The listing builds one solid part. Answer for the finished solid, in the listing's coordinates (mm). Face numbers are marked on the shaded views. A direction names the side the tool comes from. Coordinates: 2 decimals unless noted, no trailing zeros. Write each loop counter-clockwise with the first axis right and the second up, starting at its lowest first coordinate (ties: lowest second). Pieces come first, ordered by that corner, then holes.
(1) The part is cut by section C-C on y = 1.5. Determine the outline of the cut face in (x, z).
(2) The part is cut by section B-B on x = 0. Determine the outline of the cut face in (y, z), plus the area to 3 significant figures.
(3) The part is cut by section A-A on z = 0. Determine the outline of the cut face in (x, y), plus the area to 3 significant figures.
(4) Straight lines are drawn through the part: line 1 (Z direction, x = 28, y = -2.25); line 2 (Z direction, x = -23, y = 1.45); line 3 (Y direction, x = 26.5, z = 0.5). For each, find the intervals that lie inside material, in ascending order.
(5) The part is cut by section D-D on x = 24. Determine the outline of the cut face in (y, z) (3 decimals).
(6) Which of the six approach directions +Z, -Z, +X, -X, +Y, -Y give full straight-line access (tool end or side, diameter ignored) to the marked faces 1 and 2?
(7) Given P1, Ø1, axis at x = -18, z = 14, coming from the -Y side, flat-ended and moving along its own axis, determine where the tip first touches the part or whether it passes through.
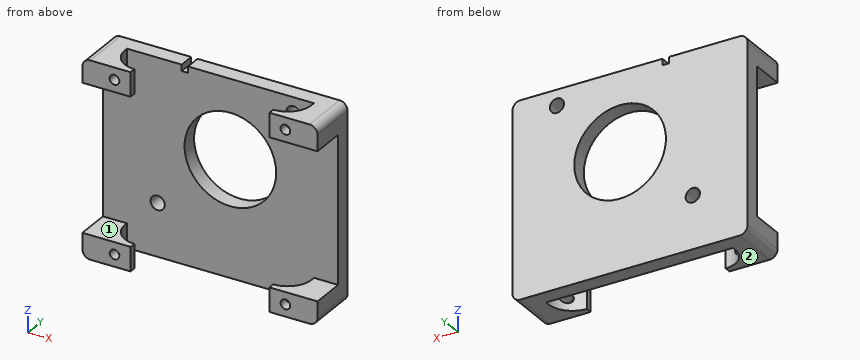
from build123d import *

# Parameters (mm, degrees)
SKETCH1_R           = 14.5
SKETCH1_R_2         = 2.25
BOSS_EXTRUDE1_DEPTH = 5
SKETCH2_W           = 7.62
SKETCH2_H           = 7.62
BOSS_EXTRUDE2_DEPTH = 10.795
SKETCH4_W           = 7.62
SKETCH4_H           = 7.62
SKETCH4_R           = 1.524
BOSS_EXTRUDE3_DEPTH = 2
BOSS_EXTRUDE4_START = -7.62
BOSS_EXTRUDE4_DEPTH = 7.62
BOSS_EXTRUDE5_START = -7.62
BOSS_EXTRUDE5_DEPTH = 7.62
SKETCH4_2_R         = 1.524
CUT_EXTRUDE1_DEPTH  = 10.795
FILLET1_R           = 2.54


with BuildPart() as part:
    # Sketch1 → Boss-Extrude1 (new body)
    with BuildSketch(Plane(origin=(0, 0, 0), x_dir=(1, 0, 0), z_dir=(0, 1, 0))):
        Polygon((-40.324, -25), (-15.4, -25), (-15.4, -23), (-13.4, -23), (-13.4, -25), (34.098, -25), (34.098, 36.722), (-40.324, 36.722), align=None)
        Circle(SKETCH1_R, mode=Mode.SUBTRACT)
        with Locations((-23, 20)):
            Circle(SKETCH1_R_2, mode=Mode.SUBTRACT)
        with Locations((20, -20)):
            Circle(SKETCH1_R_2, mode=Mode.SUBTRACT)
    extrude(amount=BOSS_EXTRUDE1_DEPTH)

    # Sketch2 → Boss-Extrude2 (add)
    with BuildSketch(Plane.XZ):
        with Locations((-36.514, 21.19)):
            Rectangle(SKETCH2_W, SKETCH2_H)
        with Locations((30.288, 21.19)):
            Rectangle(SKETCH2_W, SKETCH2_H)
        with Locations((30.288, -32.912)):
            Rectangle(SKETCH2_W, SKETCH2_H)
        with Locations((-36.514, -32.912)):
            Rectangle(SKETCH2_W, SKETCH2_H)
    extrude(amount=BOSS_EXTRUDE2_DEPTH)

    # Sketch4 → Boss-Extrude3 (add)
    with BuildSketch(Plane.XZ.offset(10.795)):
        with Locations((-28.894, 21.19)):
            Rectangle(SKETCH4_W, SKETCH4_H)
        with Locations((-30.164, 21.19)):
            Circle(SKETCH4_R, mode=Mode.SUBTRACT)
        with Locations((-28.894, -32.912)):
            Rectangle(SKETCH4_W, SKETCH4_H)
        with Locations((-30.164, -32.912)):
            Circle(SKETCH4_R, mode=Mode.SUBTRACT)
        with Locations((22.668, -32.912)):
            Rectangle(SKETCH4_W, SKETCH4_H)
        with Locations((23.938, -32.912)):
            Circle(SKETCH4_R, mode=Mode.SUBTRACT)
        with Locations((22.668, 21.19)):
            Rectangle(SKETCH4_W, SKETCH4_H)
        with Locations((23.938, 21.19)):
            Circle(SKETCH4_R, mode=Mode.SUBTRACT)
    extrude(amount=-BOSS_EXTRUDE3_DEPTH)

    # Sketch5 → Boss-Extrude4 (add)
    with BuildSketch(Plane.XY.offset(25).offset(BOSS_EXTRUDE4_START)):
        with BuildLine():
            Line((-25.084, -8.795), (-32.704, -8.795))
            Line((-32.704, -8.795), (-32.704, -1.175))
            ThreePointArc((-32.704, -1.175), (-30.472153673, -6.563153673), (-25.084, -8.795))
        make_face()
        with BuildLine():
            Line((18.858, -8.795), (26.478, -8.795))
            Line((26.478, -8.795), (26.478, -1.175))
            ThreePointArc((26.478, -1.175), (24.246153673, -6.563153673), (18.858, -8.795))
        make_face()
    extrude(amount=BOSS_EXTRUDE4_DEPTH)

    # Sketch6 → Boss-Extrude5 (add)
    with BuildSketch(Plane(origin=(0, 0, -36.722), x_dir=(-1, 0, 0), z_dir=(0, 0, -1)).offset(BOSS_EXTRUDE5_START)):
        with BuildLine():
            Line((-26.478, -8.795), (-26.478, -1.175))
            ThreePointArc((-26.478, -1.175), (-24.246153673, -6.563153673), (-18.858, -8.795))
            Line((-18.858, -8.795), (-26.478, -8.795))
        make_face()
        with BuildLine():
            Line((32.704, -8.795), (32.704, -1.175))
            ThreePointArc((32.704, -1.175), (30.472153673, -6.563153673), (25.084, -8.795))
            Line((25.084, -8.795), (32.704, -8.795))
        make_face()
    extrude(amount=BOSS_EXTRUDE5_DEPTH)

    # Sketch4<2> → Cut-Extrude1 (cut)
    with BuildSketch(Plane.XZ.offset(10.795)):
        with Locations((23.938, 21.19)):
            Circle(SKETCH4_2_R)
        with Locations((-30.164, -32.912)):
            Circle(SKETCH4_2_R)
        with Locations((-30.164, 21.19)):
            Circle(SKETCH4_2_R)
        with Locations((23.938, -32.912)):
            Circle(SKETCH4_2_R)
    extrude(amount=-CUT_EXTRUDE1_DEPTH, mode=Mode.SUBTRACT)

    # Fillet1
    fillet1_edges = [part.edges().sort_by_distance(p)[0] for p in [
        (-40.324, -2.8975, 25),
        (-40.324, -2.8975, -36.722),
        (34.098, -2.8975, -36.722),
        (34.098, -2.8975, 25),
    ]]
    fillet(fillet1_edges, radius=FILLET1_R)


solid = part.part
Model answer:
1. outline: (-40.32, -34.18) arc R2.54 ccw to (-37.78, -36.72) - (31.56, -36.72) arc R2.54 ccw to (34.1, -34.18) - (34.1, 22.46) arc R2.54 ccw to (31.56, 25) - (-13.4, 25) - (-13.4, 23) - (-15.4, 23) - (-15.4, 25) - (-37.78, 25) arc R2.54 ccw to (-40.32, 22.46) - close; hole circle Ø4.5 at (-23, -20); hole circle Ø29 at (0, 0); hole circle Ø4.5 at (20, 20)
2. outline: (0, -36.72) - (5, -36.72) - (5, -14.5) - (0, -14.5) - close; (0, 14.5) - (5, 14.5) - (5, 25) - (0, 25) - close
2. area: 164 mm2
3. outline: (-40.32, 0) - (-14.5, 0) - (-14.5, 5) - (-40.32, 5) - close; (14.5, 0) - (34.1, 0) - (34.1, 5) - (14.5, 5) - close
3. area: 227 mm2
4. line 1: z = -36.72 to -29.1, 17.38 to 25
4. line 2: z = -36.72 to -22.25, -17.75 to 25
4. line 3: y = 0 to 5
5. outline: (-10.795, -36.722) - (-6.799, -36.722) - (-6.799, -34.435) - (-10.795, -34.435) - close; (-10.795, -31.389) - (-6.799, -31.389) - (-6.799, -29.102) - (-10.795, -29.102) - close; (-10.795, 17.38) - (-6.799, 17.38) - (-6.799, 19.667) - (-10.795, 19.667) - close; (-10.795, 22.713) - (-6.799, 22.713) - (-6.799, 25) - (-10.795, 25) - close; (0, -36.722) - (5, -36.722) - (5, 25) - (0, 25) - close
6. face 1: +X, -X, -Y
6. face 2: -Z, +X, -X, +Y, -Y
7. P1: stops at y = 0
